Read the model definition and answer for the solid it produces. Units are mm, in the model's axes. Face numbers are marked on the shaded views. A direction names the side the tool comes from. Coordinates: 2 decimals unless noted, no trailing zeros. Loops run counter-clockwise (first coordinate to the right, second up) from the corner with the lowest first, then second, coordinate; pieces in that order, holes last.
Q1. Straight lines are drawn through the part: line 1 (Z direction, x = 4, y = 4.1); line 2 (X direction, y = 2.3, z = -4.25); line 3 (Z direction, x = 3.5, y = 2.3). For each, find the intervals that lie inside material, in ascending order.
Q2. The mould has two halves that part along Y. Classify the marked faces 1, 2, 3 and 4: pulls with the +Y half, pulls with the -Y half, needs draft (parallel to the pull), parting line crosses it, or undercut.
Q3. Flat-ended cylindrical pins translate along their axes: P1, Ø1.2, axis at y = 1.5, z = -4.5, coming from the +X side; P2, Ø0.6, axis at y = 4, z = -5, coming from the -X side; P3, Ø1.6, axis at x = 6, z = -1.5, coming from the -Y side. Find the tip coordinate at first contact, or state that the pin passes through.
Q4. Section C-C (y = 2.25) is taken. Count the separate pieces of the cut face and the enclosed holes in it, then the cut area to 3 significant figures.
Q5. Section A-A (x = 3.5) is taken. Give the vertices of the cut face in (y, z), then the cut area to 4 significant figures.
Q6. Section D-D (x = 8.75) is taken. Give the vertices of the cut face in (y, z).
Q7. Which of the six approach directions +Z, -Z, +X, -X, +Y, -Y give full straight-line access (tool end or side, diameter ignored) to the marked faces 5, 6, 7, 8 and 9?
Q8. Section B-B (z = 1.5) is taken. Give the vertices of the cut face in (x, y), then the cut area to 3 significant figures.
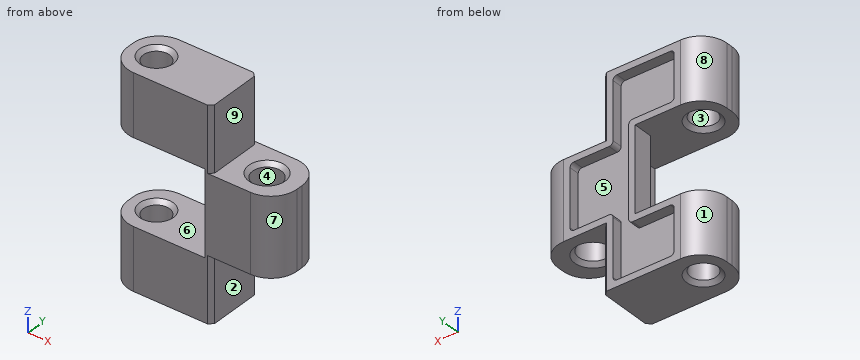
from build123d import *

# Parameters (mm, degrees)
GRUNDK_RPER_DEPTH         = 4.5
ACHSBOHHRUNGEN_DEPTH      = 16.913830463
ACHSBOHHRUNGEN_DEPTH_BACK = 16.913830463
SKIZZE2_R                 = 1
SKIZZE2_R_2               = 1.1
SKIZZE3_W                 = 2
SKIZZE3_H                 = 6.5
AUSSCHNITT_ZAHN_DEPTH     = 3
VERRUNDUNG2_R             = 2
FASE1_SIZE                = 0.3
FASE2_SIZE                = 0.3
MOOSGUMMIVERTIEFUNG_DEPTH = 0.8
VERRUNDUNG8_R             = 0.3


with BuildPart() as part:
    # Skizze1 → Grundkörper (new body)
    with BuildSketch(Plane(origin=(0, 0, 0), x_dir=(1, 0, 0), z_dir=(0, 1, 0))):
        Polygon((5.5, 3.25), (5.5, -3.25), (0, -3.25), (0, -8), (8, -8), (8, -3), (13, -3), (13, 3), (8, 3), (8, 8), (0, 8), (0, 3.25), align=None)
    extrude(amount=GRUNDK_RPER_DEPTH)

    # Skizze2 → Achsbohhrungen (cut, two sides: drawn at the far end of the back side and taken through both)
    with BuildSketch(Plane.XY.offset(-ACHSBOHHRUNGEN_DEPTH_BACK)):
        with Locations((2, 2.25)):
            Circle(SKIZZE2_R)
        with Locations((10.5, 2.25)):
            Circle(SKIZZE2_R_2)
    extrude(amount=ACHSBOHHRUNGEN_DEPTH + ACHSBOHHRUNGEN_DEPTH_BACK, mode=Mode.SUBTRACT)

    # Skizze3 → Ausschnitt Zahn (cut)
    with BuildSketch(Plane.XZ):
        with Locations((6.5, 0)):
            Rectangle(SKIZZE3_W, SKIZZE3_H)
    extrude(amount=-AUSSCHNITT_ZAHN_DEPTH, mode=Mode.SUBTRACT)

    # Verrundung2
    verrundung2_edges = [part.edges().sort_by_distance(p)[0] for p in [
        (0, 0, -5.625),
        (13, 0, 0),
        (0, 0, 5.625),
        (13, 4.5, 0),
        (0, 4.5, -5.625),
        (0, 4.5, 5.625),
    ]]
    fillet(verrundung2_edges, radius=VERRUNDUNG2_R)

    # Fase1
    fase1_edges = [part.edges().sort_by_distance(p)[0] for p in [
        (8, 0, -5.5),
        (8, 4.5, 5.5),
        (8, 0, 5.5),
        (8, 4.5, -5.5),
    ]]
    chamfer(fase1_edges, length=FASE1_SIZE)

    # Fase2
    fase2_edges = [part.edges().sort_by_distance(p)[0] for p in [
        (1, 2.25, 3.25),
        (1, 2.25, -8),
        (1, 2.25, -3.25),
        (1, 2.25, 8),
        (9.4, 2.25, -3),
        (9.4, 2.25, 3),
    ]]
    chamfer(fase2_edges, length=FASE2_SIZE)

    # Skizze6 → MoosgummiVertiefung (cut)
    with BuildSketch(Plane(origin=(0, 4.5, 0), x_dir=(1, 0, 0), z_dir=(0, 1, 0))):
        Polygon((10.5, -2.5), (10.5, 2.5), (7.2, 2.5), (7.2, 7.5), (2.5, 7.5), (2.5, 3.75), (6, 3.75), (6, -3.75), (2.5, -3.75), (2.5, -7.5), (7.2, -7.5), (7.2, -2.5), align=None)
    extrude(amount=-MOOSGUMMIVERTIEFUNG_DEPTH, mode=Mode.SUBTRACT)

    # Verrundung8
    verrundung8_edges = [part.edges().sort_by_distance(p)[0] for p in [
        (10.5, 4.1, 2.5),
        (7.2, 4.1, 2.5),
        (7.2, 4.1, 7.5),
        (2.5, 4.1, 7.5),
        (2.5, 4.1, 3.75),
        (6, 4.1, 3.75),
        (6, 4.1, -3.75),
        (2.5, 4.1, -3.75),
        (2.5, 4.1, -7.5),
        (7.2, 4.1, -7.5),
        (7.2, 4.1, -2.5),
        (10.5, 4.1, -2.5),
    ]]
    fillet(verrundung8_edges, radius=VERRUNDUNG8_R)


solid = part.part
Numbers:
1. line 1: z = -8 to -7.5, -3.75 to -3.25, 3.25 to 3.75, 7.5 to 8
1. line 2: x = 0 to 1, 3 to 8
1. line 3: z = -8 to -3.25, 3.25 to 8
2. face 1: pulls with the +Y half
2. face 2: needs draft
2. face 3: undercut
2. face 4: undercut
3. P1: stops at x = 8
3. P2: stops at x = 0.4
3. P3: stops at y = 3
4. separate pieces: 4
4. enclosed holes: 0
4. area: 76.5 mm2
5. outline: (0, -8) - (4.5, -8) - (4.5, -7.5) - (3.7, -7.5) - (3.7, -3.75) - (4.5, -3.75) - (4.5, -3.25) - (0, -3.25) - close; (0, 3.25) - (4.5, 3.25) - (4.5, 3.75) - (3.7, 3.75) - (3.7, 7.5) - (4.5, 7.5) - (4.5, 8) - (0, 8) - close
5. area: 36.75 mm2
6. outline: (0, -3) - (4.5, -3) - (4.5, -2.5) - (3.7, -2.5) - (3.7, 2.5) - (4.5, 2.5) - (4.5, 3) - (0, 3) - close
7. face 5: +Y
7. face 6: -X, -Y
7. face 7: +Z, -Z, +X, -Y
7. face 8: +Z, -Z, -X, +Y
7. face 9: +Z, +X, +Y, -Y
8. outline: (5.5, 3) - (7.5, 3) - (7.5, 0) - (11, 0) arc R2 ccw to (13, 2) - (13, 2.5) arc R2 ccw to (11, 4.5) - (10.5, 4.5) - (10.5, 3.7) - (6, 3.7) - (6, 4.5) - (5.5, 4.5) - close; hole circle Ø2.2 at (10.5, 2.25)
8. area: 18.6 mm2
